```python
from build123d import *

# Parameters (mm, degrees)
SKETCH1_W           = 135.975
SKETCH1_H           = 241.325
SKETCH1_W_2         = 19.425
SKETCH1_H_2         = 5.4
SKETCH1_W_3         = 5.4
SKETCH1_H_3         = 48.265
BOSS_EXTRUDE1_DEPTH = 5.4
BOSS_EXTRUDE2_DEPTH = 5.4


with BuildPart() as part:
    # Sketch1 → Boss-Extrude1 (new body)
    with BuildSketch(Plane.XY):
        Rectangle(SKETCH1_W, SKETCH1_H)
        with Locations((58.275, 123.3625)):
            Rectangle(SKETCH1_W_2, SKETCH1_H_2)
        with Locations((19.425, 123.3625)):
            Rectangle(SKETCH1_W_2, SKETCH1_H_2)
        with Locations((-19.425, 123.3625)):
            Rectangle(SKETCH1_W_2, SKETCH1_H_2)
        with Locations((-70.6875, 96.53)):
            Rectangle(SKETCH1_W_3, SKETCH1_H_3)
        with Locations((-58.275, 123.3625)):
            Rectangle(SKETCH1_W_2, SKETCH1_H_2)
        with Locations((70.6875, 48.265)):
            Rectangle(SKETCH1_W_3, SKETCH1_H_3)
        with Locations((-70.6875, 0)):
            Rectangle(SKETCH1_W_3, SKETCH1_H_3)
        with Locations((70.6875, -48.265)):
            Rectangle(SKETCH1_W_3, SKETCH1_H_3)
        with Locations((-70.6875, -96.53)):
            Rectangle(SKETCH1_W_3, SKETCH1_H_3)
        with Locations((-58.275, -123.3625)):
            Rectangle(SKETCH1_W_2, SKETCH1_H_2)
        with Locations((-19.425, -123.3625)):
            Rectangle(SKETCH1_W_2, SKETCH1_H_2)
        with Locations((19.425, -123.3625)):
            Rectangle(SKETCH1_W_2, SKETCH1_H_2)
        with Locations((58.275, -123.3625)):
            Rectangle(SKETCH1_W_2, SKETCH1_H_2)
    extrude(amount=BOSS_EXTRUDE1_DEPTH)

    # Sketch2 → Boss-Extrude2 (add)
    with BuildSketch(Plane.XY.offset(5.4)):
        Polygon((-48.52186, -120.70314), (-29.17814, -120.70314), (-29.17814, -126.10314), (-9.67186, -126.10314), (-9.67186, -120.70314), (9.67186, -120.70314), (9.67186, -126.10314), (29.17814, -126.10314), (29.17814, -120.70314), (48.52186, -120.70314), (48.52186, -126.10314), (68.02814, -126.10314), (68.02814, -72.43814), (73.42814, -72.43814), (73.42814, -24.09186), (68.02814, -24.09186), (68.02814, 24.09186), (73.42814, 24.09186), (73.42814, 72.43814), (68.02814, 72.43814), (68.02814, 126.10314), (48.52186, 126.10314), (48.52186, 120.70314), (29.17814, 120.70314), (29.17814, 126.10314), (9.67186, 126.10314), (9.67186, 120.70314), (-9.67186, 120.70314), (-9.67186, 126.10314), (-29.17814, 126.10314), (-29.17814, 120.70314), (-48.52186, 120.70314), (-48.52186, 126.10314), (-68.02814, 126.10314), (-68.02814, 120.70314), (-73.42814, 120.70314), (-73.42814, 72.35686), (-68.02814, 72.35686), (-68.02814, 24.17314), (-73.42814, 24.17314), (-73.42814, -24.17314), (-68.02814, -24.17314), (-68.02814, -72.35686), (-73.42814, -72.35686), (-73.42814, -120.70314), (-68.02814, -120.70314), (-68.02814, -126.10314), (-48.52186, -126.10314), align=None)
    extrude(amount=-BOSS_EXTRUDE2_DEPTH)


solid = part.part
```
Check sheet for the modelled part. Datum: model origin and axes. Units: mm. A direction names the side the tool comes from. Coordinates: 2 decimals unless noted, no trailing zeros. Write each loop counter-clockwise with the first axis right and the second up, starting at its lowest first coordinate (ties: lowest second). Pieces come first, ordered by that corner, then holes. Notation, with made-up numbers: M 4,-38.5 L 63,-38.5 A34 ccw 63,-2.5 Z; hole C -18,-24.75 d6. An arc over 180 degrees is marked long. Use one line per item in the form item = value.
Item 1: Sectioned sample at B-B, the plane y = -49. Record the cut outline in (x, z), and give its area (3 significant figures).
Answer below:
outline = M -68.03,0 L 73.43,0 L 73.43,5.4 L -68.03,5.4 Z
area = 764 mm^2
Item 2: Set-up check for faces 1 (the face through (29.178, -123, 3)), 2 (the face through (71, -72.438, 3)), 3 (the face through (-9.672, 123, 3)), 4 (the face through (68.028, 99, 3)), 5 (the face through (-68.028, 123, 3)): record each of +Z, -Z, +X, -X, +Y, -Y from which the full face is reachable in a straight line by a thin tool's end or side.
Answer below:
face_1 = +Z, -Z, -Y
face_2 = +Z, -Z, +X, -Y
face_3 = +Z, -Z, +Y
face_4 = +Z, -Z, +X, +Y
face_5 = +Z, -Z, -X, +Y
Item 3: Material ranges on L1, parallel to X at y = -78.5, z = 4.6; L2, parallel to Y at x = -4.5, z = 0.95; L3, parallel to X at y = -38, z = 0.5, recorded low to high. Write a range as from..to.
Answer below:
L1 = -73.43..68.03
L2 = -120.7..120.7
L3 = -68.03..73.43
Item 4: Release check for a two-part mould opening along X. For faces 6 (the face through (-20, -126.103, 3)), 7 (the face through (-39, -120.703, 3)), 8 (the face through (68.028, -100, 3)), 9 (the face through (9.672, 123, 3)) record: pulls with the +X half, pulls with the -X half, needs draft (parallel to the pull), parting line crosses it, or undercut.
Answer below:
face_6 = needs draft
face_7 = undercut
face_8 = pulls with the +X half
face_9 = undercut
Item 5: Sectioned sample at A-A, the plane x = 46. Record the cut outline in (y, z).
Answer below:
outline = M -120.7,0 L 120.7,0 L 120.7,5.4 L -120.7,5.4 Z
Item 6: Gauge pin test, flat ends, axial feed: pin 1 Ø1.6 at (y, z) = (124.5, 2.5) entering from +X; pin 2 Ø10 at (x, y) = (23.5, 1.5) entering from -Z; pin 3 Ø1.6 at (x, z) = (-70.5, 3.5) entering from +Y; pin 4 Ø1.6 at (x, z) = (71.5, 1.5) entering from -Y. Record the tip position at first contact, or that the pin passes through.
Answer below:
pin_1 = 68.03
pin_2 = 0
pin_3 = 120.7
pin_4 = -72.44
